```python
from build123d import *

# Parameters (mm, degrees)
F0_W     = 66.2436261773
F0_H     = 52.6286661625
F1_DEPTH = 53.9066623896
F2_DEPTH = 53.045405075
F3_R     = 7.4993670996
F4_DEPTH = 84.1025914997


# Not quite as in the source:
# - a feature names something its author has since deleted; it is built from what else it names


with BuildPart() as f1:
    # F0 (on Front) → F1 (new body)
    with BuildSketch(Plane.XZ):
        with Locations((0.5984865129, -0.1306533813)):
            Rectangle(F0_W, F0_H)
    extrude(amount=F1_DEPTH)

    # F2 (add): a face of the model
    f2_faces = [f1.faces().sort_by_distance(p)[0] for p in [
        (0.5984865129, 0, -0.1306533813),
    ]]
    extrude(f2_faces, amount=F2_DEPTH)

    # F3 (on Right) → F4 (join)
    with BuildSketch(Plane.YZ):
        with Locations((-25.9069353342, 3.7534534931)):
            Circle(F3_R)
    extrude(amount=F4_DEPTH)


solid = f1.part
```
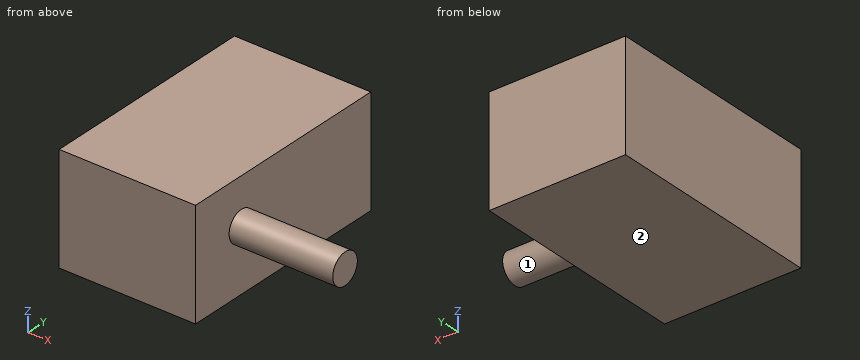
Verification items for the finished model (mm, model axes). Face numbers are marked on the shaded views. A direction names the side the tool comes from. Round coordinates to 2 decimals unless told otherwise and drop trailing zeros. Order: outer loops, then holes, each group sorted by start corner. A loop starts at its lowest first (then second) coordinate and runs counter-clockwise, first axis right, second up. Notation, with made-up numbers: (-24.5, 28.25) -> (29.5, 28.25) arc R15 ccw to (29.5, 45.25) -> close; hole circle Ø7 at (51.5, -5.5). An arc over 180 degrees is marked (long way). Put each result on its own line as item: value. Start each with the question number.
(1) Depth check by flat-ended pin: pin 1 Ø3 at (y, z) = (14.5, -0.5) entering from +X. Enter the tip coordinate at first touch or a pass-through.
(2) Section check C-C (x = 61.5). Enter the section's corners in (y, z), then the cut area to 3 significant figures.
(3) Section check B-B (y = 45.5). Enter the section's corners in (x, z).
(4) Section check D-D (z = 20.5). Enter the section's corners in (x, y), then the cut area to 3 significant figures.
(5) Material ranges on line 1 along X through (y, z) = (24.5, 1.5); line 2 along Y through (x, z) = (49, 7); line 3 along Z through (x, y) = (37, -31.5), recorded low to high.
(6) Tool access check on the marked faces 1 and 2. Record the directions out of +Z, -Z, +X, -X, +Y, -Y that give a thin tool (end or side, any length) a straight path to the whole face; none if there is none.
(7) Section check A-A (z = 2). Enter the section's corners in (x, y).
Completed:
1. pin 1: stops at x = 33.72
2. outline: circle Ø15 at (-25.91, 3.75)
2. area: 177 mm2
3. outline: (-32.52, -26.44) -> (33.72, -26.44) -> (33.72, 26.18) -> (-32.52, 26.18) -> close
4. outline: (-32.52, -53.91) -> (33.72, -53.91) -> (33.72, 53.05) -> (-32.52, 53.05) -> close
4. area: 7,080 mm2
5. line 1: x = -32.52 to 33.72
5. line 2: y = -32.67 to -19.15
5. line 3: z = -1.24 to 8.75
6. face 1: +X
6. face 2: -Z, +X, -X, +Y, -Y
7. outline: (-32.52, -53.91) -> (33.72, -53.91) -> (33.72, -33.2) -> (84.1, -33.2) -> (84.1, -18.62) -> (33.72, -18.62) -> (33.72, 53.05) -> (-32.52, 53.05) -> close
